CAD build for the part. Positions are in the model's coordinates, mm. Face numbers are marked on the shaded views. A direction names the side the tool comes from. Give positions to 0.01 mm unless a question says otherwise; leave off trailing zeros. Order: outer loops, then holes, each group sorted by start corner. A loop starts at its lowest first (then second) coordinate and runs counter-clockwise, first axis right, second up.
Item 1: Band-saw the part on D-D on z = -23.5. Give the cut face in (x, y), plus the area to 3 significant figures.
Item 2: Band-saw the part on C-C on x = 22.5. Give the cut face in (y, z).
Item 3: Two-plate mould, pull along X, no slides. Class the marked faces 3, 4, 5 and 6: released by +X, released by -X, zero draft, split by the parting line, or undercut.
Item 4: Band-saw the part on B-B on y = 80.5. Give the cut face in (x, z), plus the area to 3 significant figures.
Item 5: Which spindle directions (+Z, -Z, +X, -X, +Y, -Y) get a long thin tool onto all of the face, cutting with end or side? Do the marked faces 1 and 2. Say none if no direction does.
Item 6: Flat gauge pin, fed straight in: P1, Ø6.5, axis at x = 119.13, y = 94.765, coming from the -Z side. Where does the tip first touch, or does it go through?
Item 7: Band-saw the part on A-A on x = 119.13. Give the cut face in (y, z) (3 decimals), plus the area to 3 significant figures.
Item 8: Wall check: L1, parallel to Y at x = 6.02, z = -1.95 (3 decimals); L2, parallel to Y at x = 59.5, z = -27; L3, parallel to X at y = 46.5, z = -48. Give the ranges that are in metal, low to high.
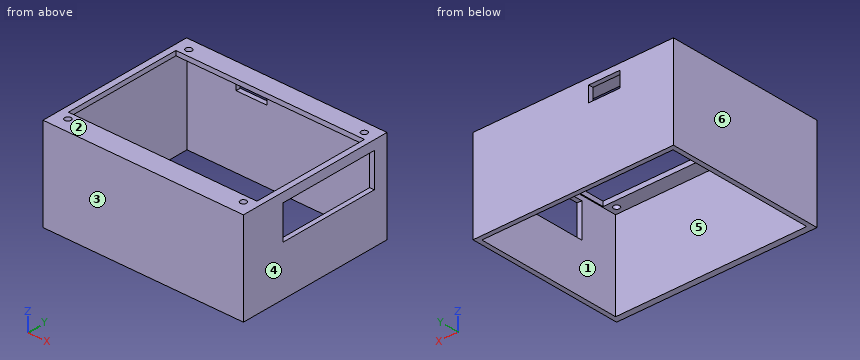
Autodesk Inventor part; units mm, degrees
ref_plane "YZ Plane" through (0, 0, 0) normal (1, 0, 0) x (0, 1, 0)
ref_plane "XZ Plane" through (0, 0, 0) normal (0, 1, 0) x (-1, 0, 0)
ref_plane "XY Plane" through (0, 0, 0) normal (0, 0, 1) x (1, 0, 0)
sketch "Sketch1" plane through (0, 0, 0) normal (0, 1, 0) x (-1, 0, 0)
  line L0 (0, 0) -> (-125.15, 0)
  line L1 (-125.15, 0) -> (-125.15, -60)
  line L2 (-125.15, -60) -> (0, -60)
  line L3 (0, -60) -> (0, 0)
  dimension "d0" = 125.15
  dimension "d1" = 60
extrude "Extrusion1" add sketch "Sketch1" along normal blind 100
sketch "Sketch2" plane through (0, 0, 0) normal (0, 0, 1) x (1, 0, 0)
  line L0 (2, 90) -> (123.51, 90)
  line L1 (123.51, 90) -> (123.51, 13.6)
  line L2 (123.51, 13.6) -> (2, 13.6)
  line L3 (2, 13.6) -> (2, 90)
  line L4 (0, 0) -> (125.15, 0)
  line L5 (0, 0) -> (0, 100)
  line L6 (0, 100) -> (125.15, 100)
  circle A0 centre (6.02, 94.765) radius 2
  circle A1 centre (6.02, 8.835) radius 2
  circle A2 centre (119.13, 94.765) radius 2
  circle A3 centre (119.13, 8.835) radius 2
  dimension "d4" = 76.4
  dimension "d5" = 121.51
  dimension "d7" = 2
  dimension "d15" = 10
  dimension "d16" = 4
  dimension "d17" = 4.765
  dimension "d18" = 4
  dimension "d19" = 85.93
  dimension "d21" = 4
  dimension "d22" = 113.11
  dimension "d23" = 6.02
  dimension "d24" = 4
  dimension "d25" = 4.765
  dimension "d26" = 113.11
extrude "Extrusion2" cut sketch "Sketch2" against normal blind 3
sketch "Sketch5" plane through (125.15, 0, 0) normal (1, 0, 0) x (0, 0, -1)
  line L0 (6, 93) -> (28, 93)
  line L1 (28, 93) -> (28, 28)
  line L2 (28, 28) -> (6, 28)
  line L3 (6, 28) -> (6, 93)
  line L4 (0, 100) -> (60, 100)
  line L5 (0, 0) -> (60, 0)
  line L6 (0, 0) -> (0, 100)
  point P0 (17, 93)
  point P1 (17, 28)
  dimension "d35" = 7
  dimension "d37" = 6
  dimension "d38" = 22
  dimension "d39" = 65
extrude "Extrusion4" cut sketch "Sketch5" against normal blind 10
sketch "Sketch7" plane through (125.15, 0, -60) normal (0, 0, -1) x (-1, 0, 0)
  line L0 (1, 99) -> (124.15, 99)
  line L1 (124.15, 99) -> (124.15, 4)
  line L2 (124.15, 4) -> (1, 4)
  line L3 (1, 4) -> (1, 99)
  line L4 (0, 100) -> (125.15, 100)
  line L5 (0, 0) -> (125.15, 0)
  line L6 (0, 0) -> (0, 100)
  line L7 (125.15, 0) -> (125.15, 100)
  dimension "d46" = 1
  dimension "d47" = 4
  dimension "d48" = 1
  dimension "d49" = 1
extrude "Extrusion6" cut sketch "Sketch7" against normal blind 57 contours L0 L1 L2 L3
sketch "Sketch8" plane through (0, 100, 0) normal (0, 1, 0) x (1, 0, 0)
  line L0 (125.15, 0) -> (125.15, 60)
  line L1 (125.15, 60) -> (0, 60)
  line L2 (125.15, 0) -> (0, 0)
  line L3 (0, 0) -> (0, 60)
  line L4 (0, 60) -> (125.15, 60)
  line L5 (125.15, 60) -> (125.15, 0)
  point P0 (0, 0)
extrude "Extrusion7" add sketch "Sketch8" along normal blind 2
sketch "Sketch9" plane through (125.15, 0, 0) normal (1, 0, 0) x (0, 0, -1)
  line L0 (0, 0) -> (60, 0)
  line L1 (0, 102) -> (60, 102)
  line L2 (60, 102) -> (60, 0)
  line L3 (60, 0) -> (0, 0)
  line L4 (0, 0) -> (0, 102)
  line L5 (6, 93) -> (28, 93)
  line L6 (28, 93) -> (28, 28)
  line L7 (6, 93) -> (28, 93)
  line L8 (28, 93) -> (28, 28)
  line L9 (28, 28) -> (6, 28)
  line L10 (6, 28) -> (6, 93)
extrude "Extrusion8" add sketch "Sketch9" along normal blind 2
sketch "Sketch10" plane through (0, 0, -60) normal (-1, 0, 0) x (0, 0, 1)
  line L0 (0, 0) -> (0, 102)
  line L1 (60, 0) -> (60, 102)
  line L2 (0, 102) -> (60, 102)
  line L3 (60, 102) -> (60, 0)
  line L4 (60, 0) -> (0, 0)
  line L5 (0, 0) -> (0, 102)
extrude "Extrusion9" add sketch "Sketch10" along normal blind 2
sketch "Sketch11" plane through (0, 102, 0) normal (0, 1, 0) x (1, 0, 0)
  line L0 (-2, 60) -> (127.15, 60)
  line L1 (62.575, 60) -> (62.575, 0)
  line L2 (-2, 0) -> (-2, 60)
  line L3 (32.575, 14) -> (52.575, 14)
  line L4 (52.575, 14) -> (52.575, 4)
  line L5 (52.575, 4) -> (32.575, 4)
  line L6 (32.575, 4) -> (32.575, 14)
  line L7 (127.15, 0) -> (-2, 0)
  point P0 (0, 0)
  dimension "d58" = 64.575
  dimension "d59" = 10
  dimension "d60" = 20
  dimension "d61" = 4
  dimension "d62" = 10
extrude "Extrusion10" cut sketch "Sketch11" against normal blind 3 contours L3 L4 L5 L6
properties part number "Behuizing_3DPrint"
The answers:
1. outline: (-2, 0) - (127.15, 0) - (127.15, 28) - (124.15, 28) - (124.15, 4) - (1, 4) - (1, 99) - (124.15, 99) - (124.15, 93) - (127.15, 93) - (127.15, 102) - (-2, 102) - close
1. area: 1,280 mm2
2. outline: (0, -60) - (4, -60) - (4, -3) - (13.6, -3) - (13.6, 0) - (0, 0) - close; (90, -3) - (99, -3) - (99, -60) - (102, -60) - (102, 0) - (90, 0) - close
3. face 3: zero draft
3. face 4: released by +X
3. face 5: undercut
3. face 6: released by -X
4. outline: (-2, -60) - (1, -60) - (1, -3) - (2, -3) - (2, 0) - (-2, 0) - close; (123.51, -3) - (124.15, -3) - (124.15, -6) - (127.15, -6) - (127.15, 0) - (123.51, 0) - close; (124.15, -60) - (127.15, -60) - (127.15, -28) - (124.15, -28) - close
4. area: 299 mm2
5. face 1: -Z
5. face 2: +Z, +X, -X, +Y, -Y
6. P1: stops at z = -3
7. outline: (0, -60) - (4, -60) - (4, -3) - (6.835, -3) - (6.835, 0) - (0, 0) - close; (10.835, -3) - (13.6, -3) - (13.6, 0) - (10.835, 0) - close; (90, -3) - (92.765, -3) - (92.765, 0) - (90, 0) - close; (96.765, -3) - (99, -3) - (99, -60) - (102, -60) - (102, 0) - (96.765, 0) - close
7. area: 452 mm2
8. L1: y = 0 to 6.835, 10.835 to 13.6, 90 to 92.765, 96.765 to 102
8. L2: y = 0 to 4, 99 to 102
8. L3: x = -2 to 1, 124.15 to 127.15
